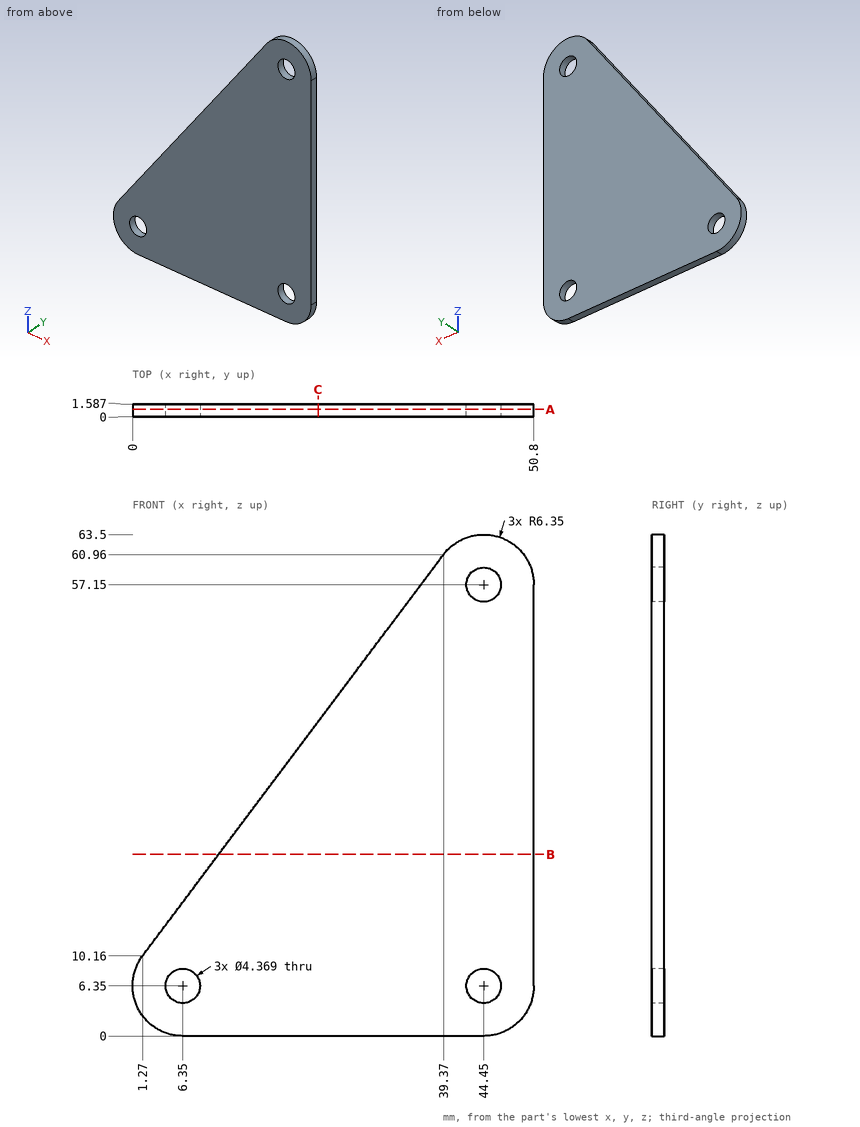
For this review, use the dimensioned drawing (mm, ordinates from the lowest corner) and the shaded views. Coordinates: 2 decimals unless noted, no trailing zeros. Order: outer loops, then holes, each group sorted by start corner. A loop starts at its lowest first (then second) coordinate and runs counter-clockwise, first axis right, second up. Notation, with made-up numbers: (-6, 50) - (10, 50) arc R24 ccw to (10, 63) - close; hole circle Ø2 at (74.25, -34.5). An arc over 180 degrees is marked (long way). Answer in a Markdown table with one row per item.
(1) Consider section A-A on y = 0.9. Give the number of separate pieces and of enclosed holes in the cut face, plus the area to 3 significant figures.
Checked values:
| item | result |
|---|---|
| separate pieces | 1 |
| enclosed holes | 3 |
| area | 2,020 mm^2 |
(2) Consider section C-C on x = 23.5. State the section outline as (y, z) points.
Checked values:
| item | result |
|---|---|
| outline | (0, 0) - (1.59, 0) - (1.59, 39.8) - (0, 39.8) - close |
(3) Consider section B-B on z = 23. State the section outline as (x, y) points.
Checked values:
| item | result |
|---|---|
| outline | (10.9, 0) - (50.8, 0) - (50.8, 1.59) - (10.9, 1.59) - close |
(4) Wall thickness on line 1 along Z through (x, y) = (44.45, 0.3) (1 decimal); line 2 along X through (y, z) = (1.25, 6) (1 decimal); line 3 along Z through (x, y) = (6.5, 0.7) (1 decimal): over which ranges is each line inside the solid? List them lowest first. Write a range as from..to.
Checked values:
| item | result |
|---|---|
| line 1 | 0..4.2, 8.5..55, 59.3..63.5 |
| line 2 | 0..4.2, 8.5..42.3, 46.6..50.8 |
| line 3 | 0..4.2, 8.5..17.1 |
(5) Clearance check with flat-ended pins moving along their axes: pin 1 (8 mm diameter, centred on x = 27, z = 46.5, fed in from -Y); pin 2 (8 mm diameter, centred on x = 13.5, z = 38, fed in from +Y). State where each tip first meets the part, or that it passes through.
Checked values:
| item | result |
|---|---|
| pin 1 | y = 0 |
| pin 2 | through |
